```python
from build123d import *

# Parameters (mm, degrees)
SKETCH_1_W          = 50
SKETCH_1_H          = 45
EXTRUDE_1_DEPTH     = 3
SKETCH_2_W          = 6
SKETCH_2_H          = 6
EXTRUDE_2_DEPTH     = 4
SKETCH_4_W          = 23
SKETCH_4_H          = 8
SKETCH_4_W_2        = 11
SKETCH_4_H_2        = 25
SKETCH_4_W_3        = 18
SKETCH_4_H_3        = 5
CUT_EXTRUDE_1_DEPTH = 4
HOLE_WIZARD_1_D     = 3


with BuildPart() as part:
    # 草图1 → 凸台-拉伸1 (new body)
    with BuildSketch(Plane(origin=(0, 0, 0), x_dir=(1, 0, 0), z_dir=(0, 1, 0))):
        Rectangle(SKETCH_1_W, SKETCH_1_H)
    extrude(amount=EXTRUDE_1_DEPTH)

    # 草图2 → 凸台-拉伸2 (add)
    with BuildSketch(Plane(origin=(0, 3, 0), x_dir=(1, 0, 0), z_dir=(0, 1, 0))):
        Polygon((22, 22.5), (15, 22.5), (2, 22.5), (2, 17.5), (15, 17.5), (15, 12.5), (22, 12.5), align=None)
        with Locations((-18, -15.5)):
            Rectangle(SKETCH_2_W, SKETCH_2_H)
        with Locations((18, -15.5)):
            Rectangle(SKETCH_2_W, SKETCH_2_H)
    extrude(amount=EXTRUDE_2_DEPTH)

    # 草图4 → 切除-拉伸1 (cut)
    with BuildSketch(Plane(origin=(0, 3, 0), x_dir=(1, 0, 0), z_dir=(0, 1, 0))):
        with Locations((-9.5, 18.5)):
            Rectangle(SKETCH_4_W, SKETCH_4_H)
        with Locations((19.5, 0)):
            Rectangle(SKETCH_4_W_2, SKETCH_4_H_2)
        with Locations((4, -20)):
            Rectangle(SKETCH_4_W_3, SKETCH_4_H_3)
    extrude(amount=-CUT_EXTRUDE_1_DEPTH, mode=Mode.SUBTRACT)

    # 孔1 (through all)
    with Locations(Plane(origin=(-17.5, 7, 15), x_dir=(0, 0, 1), z_dir=(0, 1, 0))):
        with Locations((0, 0), (0, 35), (-30, 35)):
            Hole(HOLE_WIZARD_1_D / 2)


solid = part.part
```
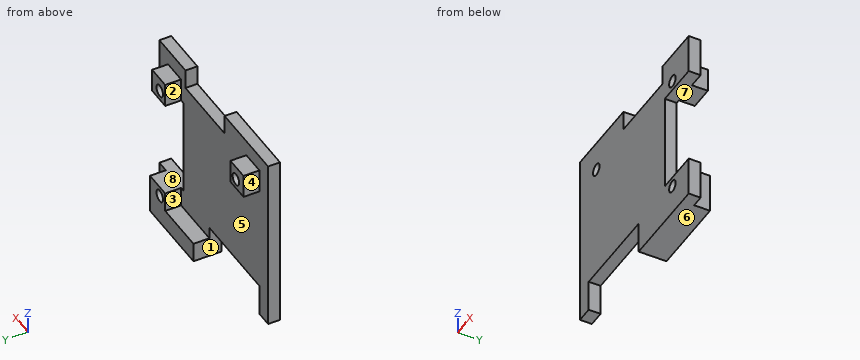
Work out the finished part from the listing and answer in its coordinate system (mm). Face numbers are marked on the shaded views. A direction names the side the tool comes from. Give positions to 0.01 mm unless a question says otherwise; leave off trailing zeros. Order: outer loops, then holes, each group sorted by start corner. A loop starts at its lowest first (then second) coordinate and runs counter-clockwise, first axis right, second up. Notation, with made-up numbers: M -33,-0.5 L -29,-0.5 A17 cw -29,3.5 Z; hole C 57.5,-12 d10. An arc over 180 degrees is marked long. Return JSON: item names as keys, results as strings.
1) Section A-A, the plane x = -17.5 is taken. Write down the section's boundary in (y, z).
Resolved:
{"outline": "M 0,-14.5 L 3,-14.5 L 3,12.5 L 7,12.5 L 7,13.5 L 0,13.5 Z; M 0,16.5 L 7,16.5 L 7,18.5 L 3,18.5 L 3,22.5 L 0,22.5 Z"}
2) A tool of negligible diameter and unlimited length cuts with its end or side. For the marked faces 1, 2, 3 and 4, from which of +Z, -Z, +X, -X, +Y, -Y can it reach the whole face along a straight path? Write none if from no direction.
Resolved:
{"face 1": "-Z, +Y, -Y", "face 2": "+Z, +Y", "face 3": "+Z, -X, +Y", "face 4": "+Z, -Z, -X, +Y"}
3) Section C-C, the plane x = 17.5 is taken. Write down the section's boundary in (y, z).
Resolved:
{"outline": "M 0,-22.5 L 7,-22.5 L 7,-16.5 L 0,-16.5 Z; M 0,-13.5 L 7,-13.5 L 7,-12.5 L 0,-12.5 Z; M 0,12.5 L 7,12.5 L 7,13.5 L 0,13.5 Z; M 0,16.5 L 7,16.5 L 7,18.5 L 3,18.5 L 3,22.5 L 0,22.5 Z"}
4) Each of these flat-tipped pins is pushed along its axis until it touches: pin 1 (22.5 mm diameter, centred on x = -10.5, z = -5.5, fed in from +Y); pin 2 (3 mm diameter, centred on x = -7.5, y = 3.5, fed in from +Z); pin 3 (4 mm diameter, centred on x = -2, y = 1, fed in from +Z); pin 4 (1.2 mm diameter, centred on x = -18.5, y = 4, fed in from +Z). Where does it stop, or does it pass through?
Resolved:
{"pin 1": "y = 3", "pin 2": "z = 22.5", "pin 3": "z = 17.5", "pin 4": "z = 18.5"}
5) Section D-D, the plane y = 2 is taken. Write down the section's boundary in (x, z).
Resolved:
{"outline": "M -25,-22.5 L -21,-22.5 L -21,-14.5 L 2,-14.5 L 2,-22.5 L 25,-22.5 L 25,-12.5 L 14,-12.5 L 14,12.5 L 25,12.5 L 25,22.5 L 13,22.5 L 13,17.5 L -5,17.5 L -5,22.5 L -25,22.5 Z; hole C -17.5,15 d3; hole C 17.5,-15 d3; hole C 17.5,15 d3"}
6) Section B-B, the plane z = 15 is taken. Write down the section's boundary in (x, y).
Resolved:
{"outline": "M -25,0 L -19,0 L -19,7 L -21,7 L -21,3 L -25,3 Z; M -16,0 L 16,0 L 16,7 L 15,7 L 15,3 L -15,3 L -15,7 L -16,7 Z; M 19,0 L 25,0 L 25,3 L 21,3 L 21,7 L 19,7 Z"}
7) For a pull along Z with two mould halves and no side action, classify the marked faces 5, 6, 7 and 8 as +Z half, -Z half, draft (parallel to the pull), parting line (faces both ways), or undercut.
Resolved:
{"face 5": "draft", "face 6": "-Z half", "face 7": "undercut", "face 8": "undercut"}
8) Straight lines are drawn through the part: line 1 along X through (y, z) = (4.75, 15); line 2 along X through (y, z) = (2.5, -15); line 3 along X through (y, z) = (3.75, -15). For each, find the intervals that lie inside material, in ascending order. Write a range as [from, to].
Resolved:
{"line 1": "[-21, -19], [-16, -15], [15, 16], [19, 21]", "line 2": "[-25, -21], [2, 16], [19, 25]", "line 3": "[15, 16], [19, 22]"}
